Work out the finished part from the listing and answer in its coordinate system (mm). Coordinates: 2 decimals unless noted, no trailing zeros. Order: outer loops, then holes, each group sorted by start corner. A loop starts at its lowest first (then second) coordinate and runs counter-clockwise, first axis right, second up. Notation, with made-up numbers: (67.5, -4) - (126.5, -4) arc R14 ccw to (126.5, 19) - close; hole circle Ø7 at (35.5, -16.5). An arc over 180 degrees is marked (long way). Answer as a JSON object with one key per item and string values. Group by question number.
1) Section A-A (y = 0) is taken. Give the vertices of the cut face in (x, z) (3 decimals).
2) Section B-B (z = 4.25) is taken. Give the vertices of the cut face in (x, y) (3 decimals), plus the area to 3 significant figures.
3) Each of these flat-tipped pins is pushed along its axis until it touches: P1, Ø5, axis at x = 84, y = 0, coming from the -Z side (3 decimals); P2, Ø3.5, axis at x = 0, y = 0, coming from the -Z side. Where does it stop, or does it pass through?
4) Find the intervals of material crossed by line 1 along Y through (x, z) = (0, 4.5) (3 decimals); line 2 along X through (y, z) = (-0.5, 7.25); line 3 along X through (y, z) = (-1, 3.75) (3 decimals), in increasing order.
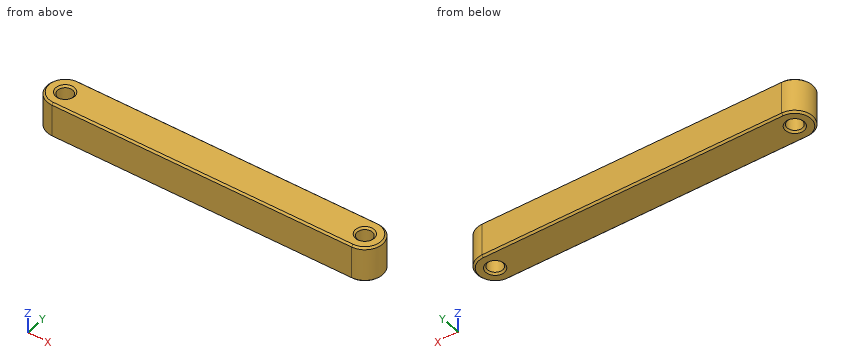
Autodesk Inventor part; units mm, degrees
ref_plane "YZ Plane" through (0, 0, 0) normal (1, 0, 0) x (0, 1, 0)
ref_plane "XZ Plane" through (0, 0, 0) normal (0, 1, 0) x (-1, 0, 0)
ref_plane "XY Plane" through (0, 0, 0) normal (0, 0, 1) x (1, 0, 0)
sketch "Sketch1" plane through (0, 0, 0) normal (0, 0, 1) x (1, 0, 0)
  circle A0 centre (0, 0) radius 2.125
  circle A1 centre (84, 0) radius 2.125
  arc A2 (84, -5) -> (84, 5) centre (84, 0) ccw
  arc A3 (0, 5) -> (0, -5) centre (0, 0) ccw
  line L0 (0, 5) -> (84, 5)
  line L1 (0, -5) -> (84, -5)
  dimension "d0" = 4.25
  dimension "d1" = 4.25
  dimension "d2" = 10
  dimension "d3" = 10
extrude "Extrusion1" add sketch "Sketch1" along normal blind 10
chamfer "Chamfer1" distance 0.5 angle 45 12 edges at (-2.125, 0, 10) (-2.125, 0, 0) (42, -5, 0) (89, 0, 0) (42, 5, 0) (-5, 0, 0) (42, -5, 10) (89, 0, 10) (42, 5, 10) (-5, 0, 10) (81.875, 0, 10) (81.875, 0, 0)
properties part number "HeightAdjustment"
Report:
{
 "1": {"outline": "(-5, 0.5) - (-4.5, 0) - (-2.625, 0) - (-2.125, 0.5) - (-2.125, 9.5) - (-2.625, 10) - (-4.5, 10) - (-5, 9.5) - close; (2.125, 0.5) - (2.625, 0) - (81.375, 0) - (81.875, 0.5) - (81.875, 9.5) - (81.375, 10) - (2.625, 10) - (2.125, 9.5) - close; (86.125, 0.5) - (86.625, 0) - (88.5, 0) - (89, 0.5) - (89, 9.5) - (88.5, 10) - (86.625, 10) - (86.125, 9.5) - close"},
 "2": {"outline": "(0, -5) - (84, -5) arc R5 ccw to (84, 5) - (0, 5) arc R5 ccw to start; hole circle Ø4.25 at (0, 0); hole circle Ø4.25 at (84, 0)", "area": "890 mm²"},
 "3": {"P1": "stops at z = 0.125", "P2": "passes through"},
 "4": {"line 1": "y = -5 to -2.125, 2.125 to 5", "line 2": "x = -4.97 to -2.07, 2.07 to 81.93, 86.07 to 88.97", "line 3": "x = -4.899 to -1.875, 1.875 to 82.125, 85.875 to 88.899"}
}
